Can you work these out from the drawing? Everything is in mm from the part's minimum corner. A direction names the side the tool comes from. Round coordinates to 2 decimals unless told otherwise and drop trailing zeros. Loops run counter-clockwise (first coordinate to the right, second up) from the corner with the lowest first, then second, coordinate; pieces in that order, holes last. Notation, with made-up numbers: (72.5, 1.5) - (125.5, 1.5) arc R12 cw to (125.5, 13.5) - close; hole circle Ø5 at (-8.75, -31). An arc over 180 degrees is marked (long way). Return JSON: item names as keys, results as strings. Group by question number.
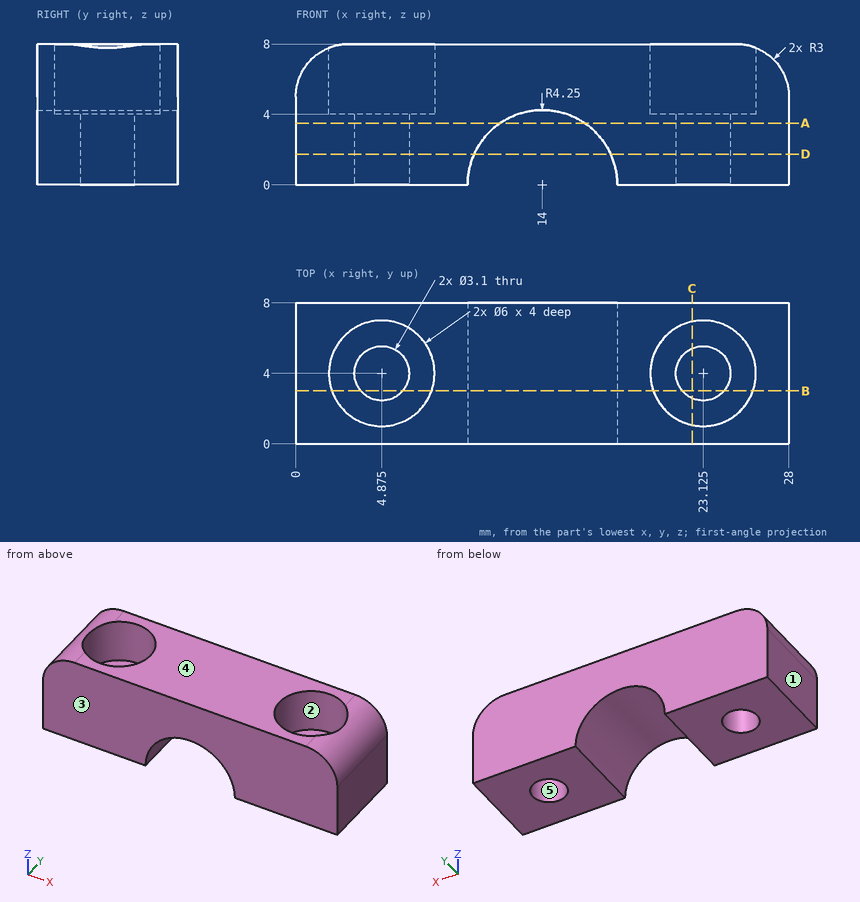
Q1. Imagine slicing it at A-A, the plane z = 3.5. List the corners of the cut face in (x, y) for me (3 decimals), and give its area (3 significant figures).
Q2. Imagine slicing it at B-B, the plane y = 3. List the corners of the cut face in (x, z) for me, and give its area (3 significant figures).
Q3. Please list where these lines run through material, in increasing order: line 1 (X direction, y = 4, z = 2.55) (3 decimals); line 2 (X direction, y = 3.75, z = 0.5); line 3 (X direction, y = 1, z = 3).
Q4. Will these pins go through, and if not, where does the flat tip stop? pin 1 Ø3 at (x, y) = (4.875, 4) entering from -Z; pin 2 Ø3 at (x, y) = (23, 4) entering from +Z.
Q5. Imagine slicing it at D-D, the plane z = 1.75. List the corners of the cut face in (x, y) for me (3 decimals), and give its area (3 significant figures).
Q6. For the marked faces 1 and 2, which set-ups out of +Z, -Z, +X, -X, +Y, -Y let a thin tool reach every point of the face, with its end or its side?
Q7. If we mould it in two halves opening along Y, with no side actions, what happens to the marked faces 3, 4 and 5? For each: +Y half, -Y half, draft (parallel to the pull), parting line (faces both ways), or undercut.
Q8. Imagine slicing it at C-C, the plane x = 22.5. List the corners of the cut face in (y, z) for me, and give its area (3 significant figures).
Output values:
{
 "1": {"outline": "(0, 0) - (11.589, 0) - (11.589, 8) - (0, 8) - close; (16.411, 0) - (28, 0) - (28, 8) - (16.411, 8) - close; hole circle Ø3.1 at (4.875, 4); hole circle Ø3.1 at (23.125, 4)", "area": "170 mm^2"},
 "2": {"outline": "(0, 0) - (3.69, 0) - (3.69, 4) - (2.05, 4) - (2.05, 7.84) arc R3 ccw to (0, 5) - close; (6.06, 0) - (9.75, 0) arc R4.25 cw to (18.25, 0) - (21.94, 0) - (21.94, 4) - (20.3, 4) - (20.3, 8) - (7.7, 8) - (7.7, 4) - (6.06, 4) - close; (24.31, 0) - (28, 0) - (28, 5) arc R3 ccw to (25.95, 7.84) - (25.95, 4) - (24.31, 4) - close", "area": "128 mm^2"},
 "3": {"line 1": "x = 0 to 3.325, 6.425 to 10.6, 17.4 to 21.575, 24.675 to 28", "line 2": "x = 0 to 3.35, 6.4 to 9.78, 18.22 to 21.6, 24.65 to 28", "line 3": "x = 0 to 10.99, 17.01 to 28"},
 "4": {"pin 1": "passes through", "pin 2": "stops at z = 4"},
 "5": {"outline": "(0, 0) - (10.127, 0) - (10.127, 8) - (0, 8) - close; (17.873, 0) - (28, 0) - (28, 8) - (17.873, 8) - close; hole circle Ø3.1 at (4.875, 4); hole circle Ø3.1 at (23.125, 4)", "area": "147 mm^2"},
 "6": {"face 1": "+Z, -Z, -X, +Y, -Y", "face 2": "+Z"},
 "7": {"face 3": "-Y half", "face 4": "draft", "face 5": "undercut"},
 "8": {"outline": "(0, 0) - (2.58, 0) - (2.58, 4) - (1.07, 4) - (1.07, 8) - (0, 8) - close; (5.42, 0) - (8, 0) - (8, 8) - (6.93, 8) - (6.93, 4) - (5.42, 4) - close", "area": "29.2 mm^2"}
}
